For this review, take the finished solid that the model builds, in its own axes (mm). A direction names the side the tool comes from. Give positions to 0.01 mm unless a question says otherwise; leave off trailing zeros. Order: outer loops, then holes, each group sorted by start corner. A loop starts at its lowest first (then second) coordinate and runs counter-clockwise, first axis right, second up.
Item 1: The part is to be moulded in two halves that separate along X. For faces 1 (the flat face through (185.574, -41.955, 3.493)), 2 (the cylindrical face through (211.866, -46.952, 1.479)), 3 (the flat face through (200, -39.5, 2)), 4 (the flat face through (219.8, -45, 2)), say which applies: released by +X, released by -X, zero draft, split by the parting line, or undercut.
Item 2: Consider section A-A (y = -45). Give the boundary of the cut face in (x, z), plus the area to 3 significant figures.
Item 3: For probe 1 along Y at (x, z) = (212.3, 1.1); probe 2 along X at (y, z) = (-46.25, 1.95); probe 3 along X at (y, z) = (-46.5, 0.6), list the stretches that pass through material, from the lowest coordinate up.
Item 4: Machinability: for faces 5 (the flat face through (200, -45, 0)), 6 (the flat face through (211, -47, 3)), which of the approach directions +Z, -Z, +X, -X, +Y, -Y give a long, thin tool a straight path to every point of the face, cutting with its end or side? Answer none if there is none.
Item 5: Consider section C-C (y = -41.5). Give the boundary of the cut face in (x, z).
Item 6: For P1, Ø2, axis at x = 186.5, y = -44, coming from the +Z side, flat-tipped, find the tip position at first contact; note if it passes through.
Item 7: Consider section B-B (z = 1.35). Give the boundary of the cut face in (x, y), plus the area to 3 significant figures.
```python
from build123d import *

# Parameters (mm, degrees)
SKETCH1_W           = 40
SKETCH1_H           = 11
SKETCH1_R           = 2
BOSS_EXTRUDE1_DEPTH = 3
SKETCH1_3_W         = 40
SKETCH1_3_H         = 11
BOSS_EXTRUDE2_DEPTH = 4


with BuildPart() as part:
    # Sketch1 → Boss-Extrude1 (new body)
    # profile 1 of 3: a face of its own
    with BuildSketch(Plane.XY):
        with Locations((199.8, -45)):
            Rectangle(SKETCH1_W, SKETCH1_H)
        Polygon((183.8, -47.020725942), (187.3, -49.041451884), (190.8, -47.020725942), (190.8, -42.979274058), (187.3, -40.958548116), (183.8, -42.979274058), align=None, mode=Mode.SUBTRACT)
        Polygon((208.8, -47.020725942), (212.3, -49.041451884), (215.8, -47.020725942), (215.8, -42.979274058), (212.3, -40.958548116), (208.8, -42.979274058), align=None, mode=Mode.SUBTRACT)
    # profile 2 of 3: a face of its own
    with BuildSketch(Plane.XY):
        Polygon((183.8, -42.979274058), (183.8, -47.020725942), (187.3, -49.041451884), (190.8, -47.020725942), (190.8, -42.979274058), (187.3, -40.958548116), align=None)
        with Locations((187.3, -45)):
            Circle(SKETCH1_R, mode=Mode.SUBTRACT)
    # profile 3 of 3: a face of its own
    with BuildSketch(Plane.XY):
        Polygon((208.8, -42.979274058), (208.8, -47.020725942), (212.3, -49.041451884), (215.8, -47.020725942), (215.8, -42.979274058), (212.3, -40.958548116), align=None)
        with Locations((212.3, -45)):
            Circle(SKETCH1_R, mode=Mode.SUBTRACT)
    extrude(amount=BOSS_EXTRUDE1_DEPTH)

    # Sketch1_3 → Boss-Extrude2 (add)
    with BuildSketch(Plane.XY):
        with Locations((199.8, -45)):
            Rectangle(SKETCH1_3_W, SKETCH1_3_H)
        Polygon((183.8, -47.020725942), (187.3, -49.041451884), (190.8, -47.020725942), (190.8, -42.979274058), (187.3, -40.958548116), (183.8, -42.979274058), align=None, mode=Mode.SUBTRACT)
        Polygon((208.8, -47.020725942), (212.3, -49.041451884), (215.8, -47.020725942), (215.8, -42.979274058), (212.3, -40.958548116), (208.8, -42.979274058), align=None, mode=Mode.SUBTRACT)
    extrude(amount=BOSS_EXTRUDE2_DEPTH)


solid = part.part
```
Resolved:
1. face 1: undercut
1. face 2: undercut
1. face 3: zero draft
1. face 4: released by +X
2. outline: (179.8, 0) - (185.3, 0) - (185.3, 3) - (183.8, 3) - (183.8, 4) - (179.8, 4) - close; (189.3, 0) - (210.3, 0) - (210.3, 3) - (208.8, 3) - (208.8, 4) - (190.8, 4) - (190.8, 3) - (189.3, 3) - close; (214.3, 0) - (219.8, 0) - (219.8, 4) - (215.8, 4) - (215.8, 3) - (214.3, 3) - close
2. area: 122 mm2
3. probe 1: y = -50.5 to -47, -43 to -39.5
3. probe 2: x = 179.8 to 185.74, 188.86 to 210.74, 213.86 to 219.8
3. probe 3: x = 179.8 to 185.98, 188.62 to 210.98, 213.62 to 219.8
4. face 5: -Z, +X, -X, +Y, -Y
4. face 6: +Z
5. outline: (179.8, 0) - (219.8, 0) - (219.8, 4) - (213.24, 4) - (213.24, 3) - (211.36, 3) - (211.36, 4) - (188.24, 4) - (188.24, 3) - (186.36, 3) - (186.36, 4) - (179.8, 4) - close
6. P1: stops at z = 3
7. outline: (179.8, -50.5) - (219.8, -50.5) - (219.8, -39.5) - (179.8, -39.5) - close; hole circle Ø4 at (187.3, -45); hole circle Ø4 at (212.3, -45)
7. area: 415 mm2
